The model under review builds one solid part; all positions refer to its coordinate system, in mm. A direction names the side the tool comes from. Coordinates: 2 decimals unless noted, no trailing zeros. Answer in a Markdown table with one row per item.
from build123d import *

# Parameters (mm, degrees)
BOSS_EXTRUDE1_DEPTH     = 50
CUT_EXTRUDE1_DEPTH      = 122
CUT_EXTRUDE1_DEPTH_BACK = 98
FILLET1_R               = 10
BOSS_EXTRUDE2_DEPTH     = 15


with BuildPart() as part:
    # Sketch1 → Boss-Extrude1 (new body)
    with BuildSketch(Plane.XY):
        with BuildLine():
            Line((112.060798049, 50), (0, 50))
            ThreePointArc((0, 50), (35.355339059, 35.355339059), (50, 0))
            ThreePointArc((50, 0), (35.355339059, -35.355339059), (0, -50))
            Line((0, -50), (112.060798049, -50))
            Line((112.060798049, -50), (112.060798049, 50))
        make_face()
    extrude(amount=BOSS_EXTRUDE1_DEPTH)

    # Sketch2 → Cut-Extrude1 (cut, two sides)
    with BuildSketch(Plane(origin=(0, 0, 0), x_dir=(1, 0, 0), z_dir=(0, 1, 0))) as cut_extrude1_sk:
        with BuildLine():
            Line((90.490413338, 0), (0, 0))
            Line((0, 0), (0, -50))
            add(Edge.make_bspline(
                [(0, -50), (54.321214116, -40.505522655), (90.490413338, 0)],
                knots=[0, 0, 0, 1, 1, 1], degree=2))
        make_face()
    extrude(amount=CUT_EXTRUDE1_DEPTH, mode=Mode.SUBTRACT)
    extrude(cut_extrude1_sk.sketch, amount=-CUT_EXTRUDE1_DEPTH_BACK, mode=Mode.SUBTRACT)

    # Fillet1
    fillet1_edges = [part.edges().sort_by_distance(p)[0] for p in [
        (90.490413338, -25, 0),
    ]]
    fillet(fillet1_edges, radius=FILLET1_R)

    # Sketch3 → Boss-Extrude2 (add)
    with BuildSketch(Plane.XY.offset(50)):
        with BuildLine():
            Line((0, 50), (61.486792526, 50))
            Line((61.486792526, 50), (61.486792526, -50))
            Line((61.486792526, -50), (0, -50))
            ThreePointArc((0, -50), (50, 0), (0, 50))
        make_face()
    extrude(amount=BOSS_EXTRUDE2_DEPTH)


solid = part.part
(1) Machinability: for faces 1 (the flat face through (103, 1, 0)), 2 (the flat face through (86, 1, 50)), which of the approach directions +Z, -Z, +X, -X, +Y, -Y give a long, thin tool a straight path to every point of the face, cutting with its end or side? Answer none if there is none.
Report:
| item | result |
|---|---|
| face 1 | -Z, +X, -X, +Y, -Y |
| face 2 | +Z, +X, +Y, -Y |
(2) Insertion check: P1, Ø1, axis at y = 38.5, z = 25.5, coming from the -X side; P2, Ø12, axis at y = 17, z = 58, coming from the +X side; P3, Ø1.5, axis at x = 95, y = -1.5, coming from the +Z side. Each pin has a flat end and moves straight along its axis. Give the tip position at first contact, or say it passes through.
Report:
| item | result |
|---|---|
| P1 | x = 60.84 |
| P2 | x = 61.49 |
| P3 | z = 50 |
(3) To check wall thickness, follow line 1 (Z direction, x = 87, y = 41); line 2 (Z direction, x = 91, y = 23); line 3 (X direction, y = 8.5, z = 38). State the ranges of each line that lie inside material, in increasing order. Write a range as [from, to].
Report:
| item | result |
|---|---|
| line 1 | [3.79, 50] |
| line 2 | [0.79, 50] |
| line 3 | [49.27, 112.06] |
